Verification items for this drawing (mm, ordinates from the low corner). A direction names the side the tool comes from. Round coordinates to 2 decimals unless told otherwise and drop trailing zeros. Order: outer loops, then holes, each group sorted by start corner. A loop starts at its lowest first (then second) coordinate and runs counter-clockwise, first axis right, second up. Notation, with made-up numbers: (89.25, -7) - (148.25, -7) arc R24 cw to (148.25, 29) - close; hole circle Ø7 at (-38.75, -28.75). An arc over 180 degrees is marked (long way). One line per question, with ' | ' between items. Start each with the question number.
Q1. Sectioned sample at C-C, the plane z = 82. Enter the section's corners in (x, y), then the cut area to 3 significant figures.
Q2. Tool access check on the marked faces 1, 2 and 3. Record the directions out of +Z, -Z, +X, -X, +Y, -Y that give a thin tool (end or side, any length) a straight path to the whole face; none if there is none.
Q3. Sectioned sample at A-A, the plane x = 101.6. Enter the section's corners in (y, z), then the cut area to 3 significant figures.
Q4. Material ranges on line 1 along Z through (x, y) = (41.5, 121); line 2 along X through (y, z) = (118.5, 83.5); line 3 along Y through (x, z) = (104.5, 26.5), recorded low to high.
Q5. Sectioned sample at D-D, the plane z = 53.5. Enter the section's corners in (x, y), then the cut area to 3 significant figures.
Q6. Gauge pin test, flat ends, axial feed: P1, Ø1, axis at y = 127.5, z = 38.5, coming from the -X side; P2, Ø3, axis at x = 141, y = 142.5, coming from the +Z side; P3, Ø1.5, axis at y = 128.5, z = 15.5, coming from the +X side. Record the tip position at first contact, or that the pin passes through.
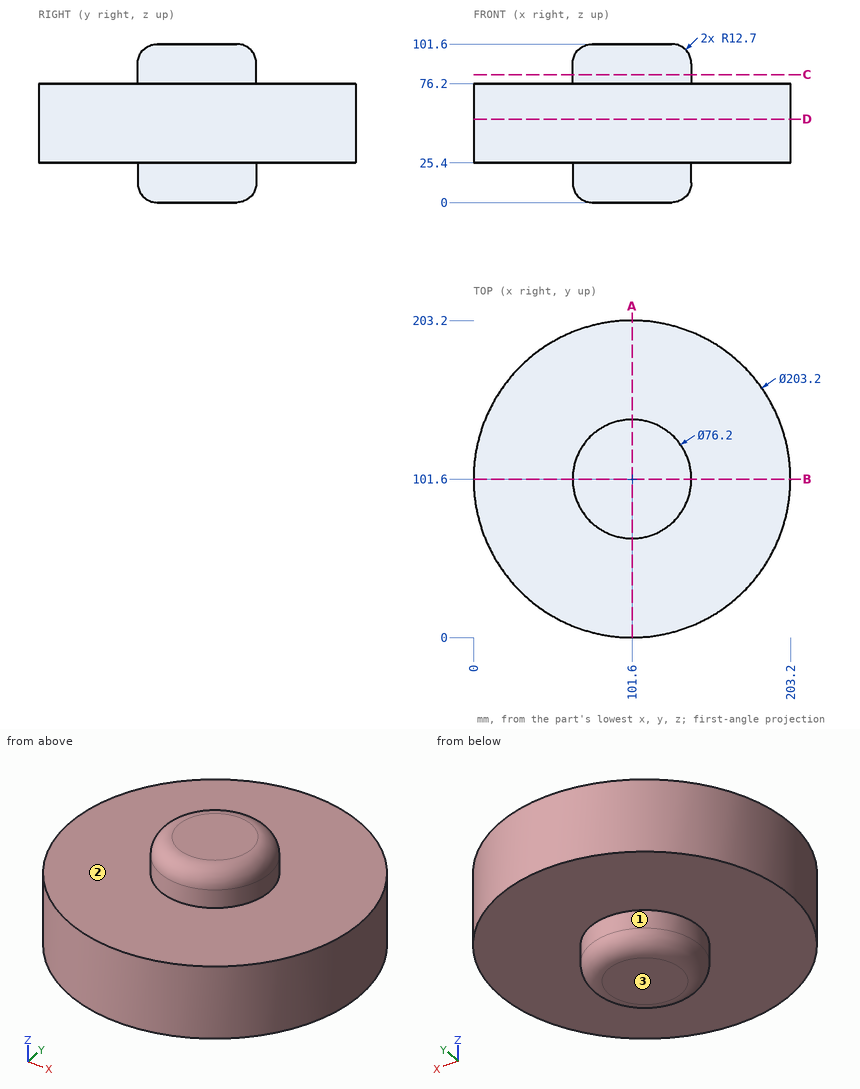
Determined:
1) outline: circle Ø76.2 at (101.6, 101.6) | area: 4,560 mm2
2) face 1: -Z | face 2: +Z | face 3: -Z, +X, -X, +Y, -Y
3) outline: (0, 25.4) - (63.5, 25.4) - (63.5, 12.7) arc R12.7 ccw to (76.2, 0) - (127, 0) arc R12.7 ccw to (139.7, 12.7) - (139.7, 25.4) - (203.2, 25.4) - (203.2, 76.2) - (139.7, 76.2) - (139.7, 88.9) arc R12.7 ccw to (127, 101.6) - (76.2, 101.6) arc R12.7 ccw to (63.5, 88.9) - (63.5, 76.2) - (0, 76.2) - close | area: 14,100 mm2
4) line 1: z = 25.4 to 76.2 | line 2: x = 67.45 to 135.75 | line 3: y = 0.04 to 203.16
5) outline: circle Ø203.2 at (101.6, 101.6) | area: 32,400 mm2
6) P1: stops at x = 3.23 | P2: stops at z = 76.2 | P3: stops at x = 129.31
